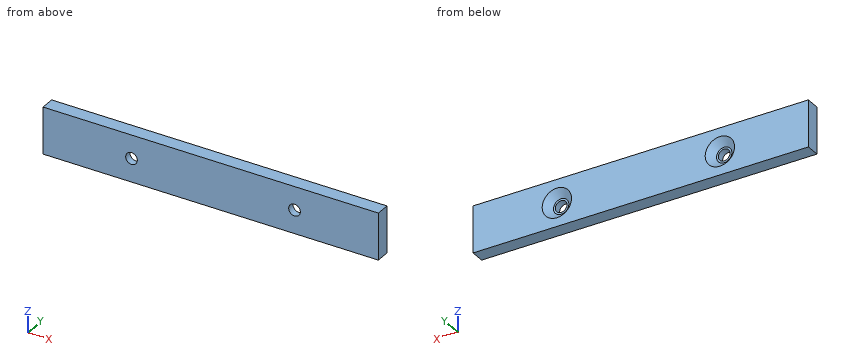
```python
from build123d import *

# Parameters (mm, degrees)
SKETCH1_W           = 144
SKETCH1_H           = 20
BOSS_EXTRUDE1_DEPTH = 6


# Read off the part's stored shape, not the designer's step: AdvancedHole1
with BuildPart() as part:
    # Sketch1 → Boss-Extrude1 (new body)
    with BuildSketch(Plane(origin=(0, 0, 0), x_dir=(1, 0, 0), z_dir=(0, 1, 0))):
        Rectangle(SKETCH1_W, SKETCH1_H)
    extrude(amount=BOSS_EXTRUDE1_DEPTH)

    # AdvancedHole1 outline → AdvancedHole1 (revolve, cut)
    with BuildSketch(Plane(origin=(36, 0, 0), x_dir=(1, 0, 0), z_dir=(0, 0, 1))):
        Polygon((0, 0), (2.5, 0), (2.5, 3), (3.3, 3), (6.3, 6), (0, 6), align=None)
    revolve(axis=Axis((36, 0, 0), (0, 1, 0)), mode=Mode.SUBTRACT)

    # AdvancedHole1 2 outline → AdvancedHole1 2 (revolve, cut)
    with BuildSketch(Plane(origin=(-34, 0, 0), x_dir=(1, 0, 0), z_dir=(0, 0, 1))):
        Polygon((6.3, 6), (0, 6), (0, 0), (2.5, 0), (2.5, 3), (3.3, 3), align=None)
    revolve(axis=Axis((-34, 0, 0), (0, 1, 0)), mode=Mode.SUBTRACT)


solid = part.part
```
Input: part model. Units: mm. Frame: model coordinates. Give positions to 0.01 mm unless a question says otherwise; leave off trailing zeros. Loops run counter-clockwise (first coordinate to the right, second up) from the corner with the lowest first, then second, coordinate; pieces in that order, holes last. Notation, with made-up numbers: (-12, -18) -> (46, -18) arc R21 cw to (46, 3) -> close; hole circle Ø8 at (20, 62). An arc over 180 degrees is marked (long way). Use a Markdown table: item, result.
Q1. First-contact query: P1, Ø8, axis at x = -34, z = 0, coming from the -Y side; P2, Ø4.5, axis at x = 36, z = 0, coming from the -Y side; P3, Ø7.5, axis at x = -33.5, z = 0, coming from the +Y side. Flat tips, straight axial feed; report the tip coordinate or a pass-through.
Entries:
| item | result |
|---|---|
| P1 | stops at y = 0 |
| P2 | passes through |
| P3 | stops at y = 3.95 |
Q2. Section query C-C, the plane y = 4.9. Return the cut outline in (x, z), plus the area to 3 significant figures.
Entries:
| item | result |
|---|---|
| outline | (-72, -10) -> (72, -10) -> (72, 10) -> (-72, 10) -> close; hole circle Ø10.4 at (-34, 0); hole circle Ø10.4 at (36, 0) |
| area | 2,710 mm² |
Q3. Section query A-A, the plane x = 36. Return the cut outline in (y, z), plus the area to 3 significant figures.
Entries:
| item | result |
|---|---|
| outline | (0, -10) -> (6, -10) -> (6, -6.3) -> (3, -3.3) -> (3, -2.5) -> (0, -2.5) -> close; (0, 2.5) -> (3, 2.5) -> (3, 3.3) -> (6, 6.3) -> (6, 10) -> (0, 10) -> close |
| area | 76.2 mm² |
Q4. Ray query, probe 1 along X at (y, z) = (0.8, 0); probe 2 along X at (y, z) = (4.95, -1.5); probe 3 along Z at (x, y) = (36, 2.2). Return the intervals inside material, ascending. Write a range as from..to.
Entries:
| item | result |
|---|---|
| probe 1 | x = -72..-36.5, -31.5..33.5, 38.5..72 |
| probe 2 | x = -72..-39.03, -28.97..30.97, 41.03..72 |
| probe 3 | z = -10..-2.5, 2.5..10 |
Q5. Section query B-B, the plane z = 0. Return the cut outline in (x, y), plus the area to 3 significant figures.
Entries:
| item | result |
|---|---|
| outline | (-72, 0) -> (-36.5, 0) -> (-36.5, 3) -> (-37.3, 3) -> (-40.3, 6) -> (-72, 6) -> close; (-31.5, 0) -> (33.5, 0) -> (33.5, 3) -> (32.7, 3) -> (29.7, 6) -> (-27.7, 6) -> (-30.7, 3) -> (-31.5, 3) -> close; (38.5, 0) -> (72, 0) -> (72, 6) -> (42.3, 6) -> (39.3, 3) -> (38.5, 3) -> close |
| area | 776 mm² |
